For this review, use the dimensioned drawing (mm, ordinates from the lowest corner) and the shaded views. A direction names the side the tool comes from. Coordinates: 2 decimals unless noted, no trailing zeros. Order: outer loops, then holes, each group sorted by start corner. A loop starts at its lowest first (then second) coordinate and runs counter-clockwise, first axis right, second up. Notation, with made-up numbers: M 71.5,-22 L 130.5,-22 A12 ccw 130.5,-6 Z; hole C 57.25,43.25 d10. An arc over 180 degrees is marked long. Use CSV: the item, a comma, the result in double quotes.
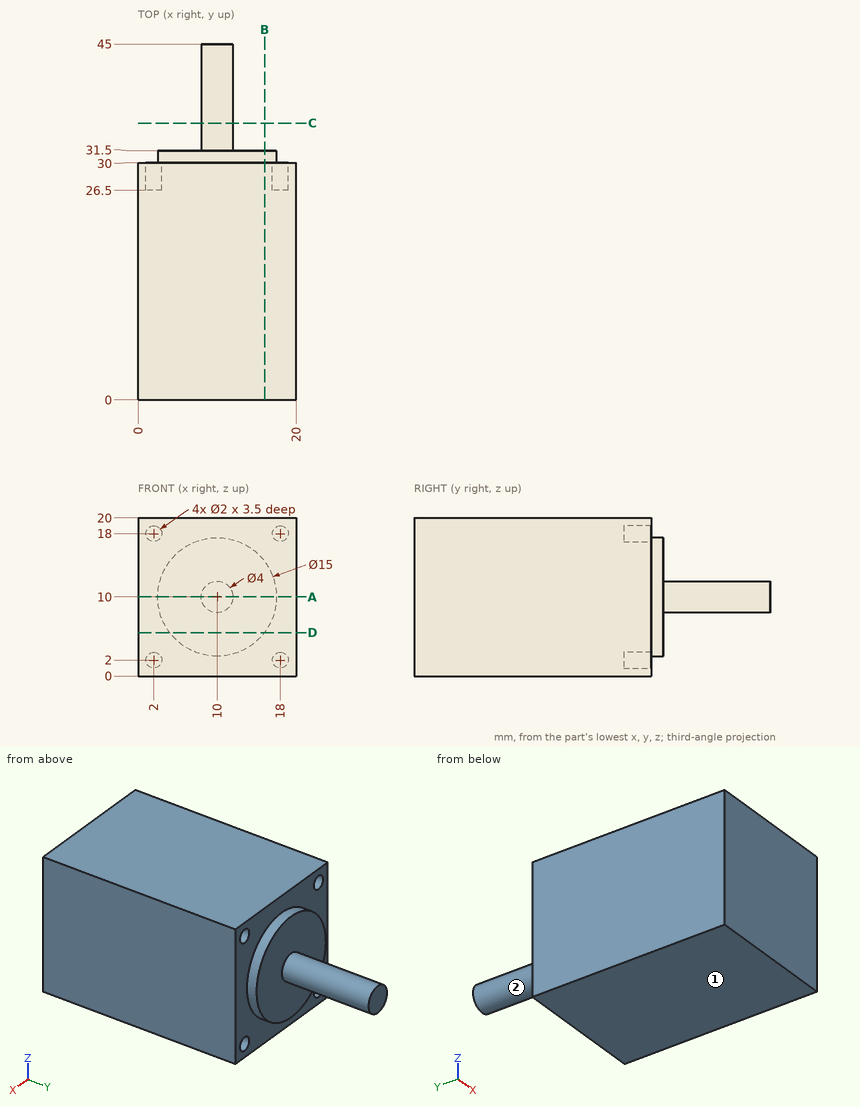
Item 1: Add section B-B on x = 16. State the section outline as (y, z) points, and give its area (4 significant figures).
Solutions:
outline,"M 0,0 L 30,0 L 30,5.5 L 31.5,5.5 L 31.5,14.5 L 30,14.5 L 30,20 L 0,20 Z"
area,"613.5 mm^2"
Item 2: For the marked faces 1 and 2, list the 3-axis set-ups (+Z, -Z, +X, -X, +Y, -Y) from which the entire face can be reached by the end or side of a thin tool; tool diameter is ignored.
Solutions:
face 1,"-Z, +X, -X, +Y, -Y"
face 2,"+Y"
Item 3: Add section D-D on z = 5.5. State the section outline as (x, y) points.
Solutions:
outline,"M 0,0 L 20,0 L 20,30 L 16,30 L 16,31.5 L 4,31.5 L 4,30 L 0,30 Z"
Item 4: Add section C-C on y = 35. State the section outline as (x, z) points, and give its area (3 significant figures).
Solutions:
outline,"C 10,10 d4"
area,"12.6 mm^2"
Item 5: To check wall thickness, follow line 1 along X through (y, z) = (28.5, 18); line 2 along Y through (x, z) = (16.75, 3); line 3 along Y through (x, z) = (7.5, 15.75). State the ranges of each line that lie inside material, in increasing order. Write a range as [from, to].
Solutions:
line 1,"[0, 1], [3, 17], [19, 20]"
line 2,"[0, 30]"
line 3,"[0, 31.5]"
Item 6: Clearance check with flat-ended pins moving along their axes: pin 1 Ø1.6 at (x, z) = (2.5, 1.5) entering from +Y; pin 2 Ø1.8 at (x, z) = (18, 18) entering from +Y; pin 3 Ø8 at (x, y) = (9.5, 40) entering from -Z. State where each tip first meets the part, or that it passes through.
Solutions:
pin 1,"y = 30"
pin 2,"y = 26.5"
pin 3,"z = 8"
Item 7: Add section A-A on z = 10. State the section outline as (x, y) points, and give its area (4 significant figures).
Solutions:
outline,"M 0,0 L 20,0 L 20,30 L 17.5,30 L 17.5,31.5 L 12,31.5 L 12,45 L 8,45 L 8,31.5 L 2.5,31.5 L 2.5,30 L 0,30 Z"
area,"676.5 mm^2"
